Can you work these out from the model? Positions are in its coordinate system, mm. A direction names the side the tool comes from. Coordinates: 2 decimals unless noted, no trailing zeros. Loops run counter-clockwise (first coordinate to the right, second up) from the corner with the lowest first, then second, coordinate; pieces in that order, holes last. Notation, with made-up numbers: (60.25, 63) - (83.25, 63) arc R31 ccw to (83.25, 90) - close; hole circle Ø8 at (0.25, 8.5). An arc over 180 degrees is marked (long way). Put each result on its own line as item: value. Start each with the question number.
Autodesk Inventor part; units mm, degrees
ref_plane "YZ Plane" through (0, 0, 0) normal (1, 0, 0) x (0, 1, 0)
ref_plane "XZ Plane" through (0, 0, 0) normal (0, 1, 0) x (-1, 0, 0)
ref_plane "XY Plane" through (0, 0, 0) normal (0, 0, 1) x (1, 0, 0)
sketch "Sketch8" plane through (0, 0, 0) normal (0, 1, 0) x (-1, 0, 0)
  circle A0 centre (0, 0) radius 38.1
  circle A1 centre (0, 0) radius 34.925
  dimension "d25" = 76.2
  dimension "d26" = 3.175
extrude "Extrusion6" add sketch "Sketch8" against normal blind 3.81 contours A0 | A1
extrude "Extrusion7" add sketch "Sketch8" along normal blind 85.09
sketch "Sketch9" plane through (0, -3.81, 0) normal (0, -1, 0) x (1, 0, 0)
  point P0 (0, 0)
sketch "Sketch10" plane through (0, 0, 0) normal (1, 0, 0) x (0, 1, 0)
  line L0 (85.09, 38.1) -> (-3.81, 38.1)
  line L1 (-3.81, 38.1) -> (-3.81, 50.8)
  line L2 (-3.81, 50.8) -> (5.715, 50.8)
  line L3 (5.715, 50.8) -> (5.715, 38.1)
  arc A0 (-0.635, 41.275) -> (-0.635, 47.625) centre (-0.635, 44.45) ccw
  line L4 (-3.81, 38.1) -> (-3.81, -38.1)
  line L5 (-0.635, 47.625) -> (-3.81, 47.625)
  line L6 (-0.635, 41.275) -> (-3.81, 41.275)
  line L7 (-16.51, 0) -> (72.39, 0)
  point P0 (0, 0)
  dimension "d31" = 6.35
  dimension "d32" = 3.175
  dimension "d35" = 3.175
  dimension "d36" = 3.175
revolve "Revolution1" add sketch "Sketch10" angle 8 mid plane about axis through (0, -10, 0) along (0, 1, 0) contours L0 L1 L6 A0 L5 L2 L3
sketch "Sketch11" plane through (0, 0, 0) normal (1, 0, 0) x (0, 1, 0)
  line L0 (85.09, 38.1) -> (5.715, 38.1)
  arc A0 (26.8199, 45.5701) -> (35.4101, 45.5701) centre (31.115, 45.5701) ccw
  line L1 (38.5851, 38.1) -> (38.5851, 53.0402)
  line L2 (23.6449, 53.0402) -> (23.6449, 38.1)
  line L3 (35.4101, 45.5701) -> (35.4101, 53.0402)
  line L4 (26.8199, 45.5701) -> (26.8199, 53.0402)
  line L5 (38.5851, 53.0402) -> (35.4101, 53.0402)
  line L6 (26.8199, 53.0402) -> (23.6449, 53.0402)
  line L7 (-16.51, 0) -> (72.39, 0)
  arc A1 (2.54, 44.45) -> (-0.635, 47.625) centre (-0.635, 44.45) ccw
  arc A2 (-0.635, 41.275) -> (2.54, 44.45) centre (-0.635, 44.45) ccw
  point P0 (0, 0)
  dimension "d38" = 8.5902
  dimension "d39" = 3.175
  dimension "d40" = 3.175
  dimension "d41" = 3.175
  dimension "d44" = 31.75
revolve "Revolution2" add sketch "Sketch11" angle 10 mid plane about axis through (0, -10, 0) along (0, 1, 0)
pattern_circular "Circular Pattern2" count 3 over 90 about axis through (0, -10, 0) along (0, 1, 0) of "Revolution2", "Revolution1"
equation "\"d25\" = outerDiameter"
equation "\"d26\" = wallThickness"
equation "\"d27\" = floorThickness"
equation "\"d29\" = height - floorThickness"
equation "\"d31\" = holeDiameter"
equation "\"d32\" = fromWallToHole"
equation "\"d35\" = fromEdgeToWall"
equation "\"d36\" = htAboveHole"
equation "\"d39\" = fromWallToHole"
equation "\"d40\" = htAboveHole"
equation "\"d41\" = htAboveHole"
equation "\"d44\" = spaceBetweenWire"
equation "\"htAboveHole\" = 3.175"
equation "\"fromWallToHole\" = 3.175"
equation "\"fromEdgeToWall\" = 3.175"
equation "\"holeDiameter\" = 6.35"
equation "\"bottomHeight\" = holeDiameter + htAboveHole"
equation "\"d42\" = fromEdgeToWall"
equation "\"outerDiameter\" = 76.2"
equation "\"floorThickness\" = 3.81"
equation "\"wallThickness\" = 3.175"
equation "\"spaceBetweenWire\" = 31.75"
equation "\"height\" = 88.9"
properties part number "roundMouseSupport"
Q1. I want a section at B-B on y = 10. List the corners of the cut face in (x, z) for me (3 decimals).
Q2. Will these pins go through, and if not, where does the flat tip stop? pin 1 (10 mm diameter, centred on x = 27, y = 59.5, fed in from +Z); pin 2 (3.5 mm diameter, centred on x = 0, z = 44.5, fed in from +Y); pin 3 (4 mm diameter, centred on y = 7.5, z = -5.5, fed in from +X).
Q3. I want a section at C-C on z = 0. List the corners of the cut face in (x, y) for me (3 decimals), and give its area (3 significant figures).
Q4. I want a section at A-A on x = 0. List the corners of the cut face in (y, z) for me (3 decimals), and give its area (3 significant figures).
Q5. We'd pull the mould along X, two halves only. Please class faces 1 (the flat face through (49, -3.81, 0)), 2 (the cylindrical face through (47.625, -2.245, -0.047)), 3 (the flat face through (40.54, 31.01, -3.547)), 4 (the cylindrical face through (0.04, -2.245, 41.275)): released by +X, released by -X, zero draft, split by the parting line, or undercut.
Q6. I want a section at D-D on z = 44. Count the separate pieces of the cut face and the enclosed holes in it, and give its area (3 significant figures).
Q7. On a 3-axis mill with a long thin cutter (end or side, diameter ignored), from which of +Z, -Z, +X, -X, +Y, -Y can I reach the whole of each face in a straight line? I mean faces 5 (the flat face through (31.174, 31.01, 26.158)), 6 (the flat face through (35, 26.82, 34)), 7 (the flat face through (0, 5.715, 44)). Say none if no direction works.
Q8. Please list where these lines run through material, in increasing order: line 1 along Z through (x, y) = (0, 52) (3 decimals); line 2 along X through (y, z) = (49.5, -25.5); line 3 along X through (y, z) = (24, -13.5). Write a range as [from, to].
Calculated:
1. outline: circle Ø76.2 at (0, 0); hole circle Ø69.85 at (0, 0)
2. pin 1: z = 31.11
2. pin 2: y = 38.59
2. pin 3: x = 37.94
3. outline: (-38.1, -3.81) - (41.275, -3.81) - (41.275, -0.635) arc R3.175 cw to (47.625, -0.635) - (47.625, -3.81) - (50.8, -3.81) - (50.8, 5.715) - (38.1, 5.715) - (38.1, 23.645) - (53.04, 23.645) - (53.04, 26.82) - (45.57, 26.82) arc R4.295 cw to (45.57, 35.41) - (53.04, 35.41) - (53.04, 38.585) - (38.1, 38.585) - (38.1, 85.09) - (34.925, 85.09) - (34.925, 0) - (-34.925, 0) - (-34.925, 85.09) - (-38.1, 85.09) - close
3. area: 1,050 mm2
4. outline: (-3.81, -38.1) - (85.09, -38.1) - (85.09, -34.925) - (0, -34.925) - (0, 34.925) - (85.09, 34.925) - (85.09, 38.1) - (38.585, 38.1) - (38.585, 53.04) - (35.41, 53.04) - (35.41, 45.57) arc R4.295 cw to (26.82, 45.57) - (26.82, 53.04) - (23.645, 53.04) - (23.645, 38.1) - (5.715, 38.1) - (5.715, 50.8) - (-3.81, 50.8) - (-3.81, 47.625) - (-0.635, 47.625) arc R3.175 cw to (-0.635, 41.275) - (-3.81, 41.275) - close
4. area: 1,050 mm2
5. face 1: zero draft
5. face 2: undercut
5. face 3: undercut
5. face 4: split by the parting line
6. separate pieces: 3
6. enclosed holes: 0
6. area: 72.8 mm2
7. face 5: +X, +Y, -Y
7. face 6: +Z, +X
7. face 7: +Z, +X, -X
8. line 1: [-38.1, -34.925], [34.925, 38.1]
8. line 2: [-28.31, -23.86], [23.86, 28.31]
8. line 3: [-35.63, -32.21], [32.21, 35.63]
